Input: part model. Units: mm. Frame: model coordinates. A direction names the side the tool comes from. Give positions to 0.01 mm unless a question says otherwise; leave off trailing zeros. Loops run counter-clockwise (first coordinate to the right, second up) from the corner with the lowest first, then second, coordinate; pieces in that order, holes last. Notation, with made-up numbers: M 23.25,-15.5 L 28.25,-15.5 A20 ccw 28.25,5.5 Z; hole C -30.75,48 d11. An arc over 180 degrees is marked long. One line per item, written item: value. Start each with the question number.
(1) Pull-direction query (X, two-part tool) for faces 1 (the conical face through (26.98, -24.99, 7.22)), 2 (the flat face through (14, 23, 8)), 3 (the conical face through (13.95, 21.71, -9.38)); classes: released by +X, released by -X, zero draft, split by the parting line, or undercut.
(2) Ray query, line 1 along X through (y, z) = (-25.1, 12); line 2 along Y through (x, z) = (14.5, 13.5); line 3 along Y through (x, z) = (31, 12). Return the intervals inside material, ascending. Write a range as from..to.
(3) Section B-B on y = 0. Output: boundary loops of the cut face in (x, z).
(4) Pin query (flat end, axial travel): P1, Ø4, axis at x = 14, y = 21.5, coming from the -Z side; P2, Ø5.5, axis at y = -9.53, z = 5.5, coming from the -X side; P3, Ø4, axis at x = 6.5, y = -18, coming from the -Z side. Return the tip coordinate at first contact, or that it passes through.
(5) Section C-C on x = 22. State how many separate pieces and enclosed holes the cut face has, plus the area to 3 significant figures.
(6) Access query for faces 4 (the cylindrical face through (14.921, 20.655, -15.057)), 5 (the flat face through (16, -25, -18)), 6 (the cylindrical face through (14.1, -0.506, -22.994)). Directions: +Z, -Z, +X, -X, +Y, -Y. A direction counts if a zero-diameter tool reaches every point of the face in a straight line with its end or side. Return the directions, or none.
(7) Section A-A on z = -4. Output: boundary loops of the cut face in (x, y).
(8) Section D-D on y = -15.5. Output: boundary loops of the cut face in (x, z), plus the area to 3 significant figures.
```python
from build123d import *

# Parameters (mm, degrees)
MOTOR_SHELL_DEPTH               = 32.6
MOTOR_MOUNT_DEPTH               = 4
MOUNTING_HOLE_D                 = 3.4
MOUNTING_HOLE_CSINK_D           = 6.72
MOUNTING_HOLE_CSINK_ANGLE       = 90
HOLE_DUPLICATION_COUNT          = 3
SKETCH11_R                      = 6.5
SHAFT_BASE_CUTOUT_DEPTH         = 33.6
M3X0_5_TAPPED_HOLE1_D           = 2.5
M3X0_5_TAPPED_HOLE1_DEPTH       = 5
M3X0_5_TAPPED_HOLE1_CSINK_D     = 3.05
M3X0_5_TAPPED_HOLE1_CSINK_ANGLE = 90
M3X0_5_TAPPED_HOLE1_TIP         = 0.751075774
M3X0_5_TAPPED_HOLE2_D           = 2.5
M3X0_5_TAPPED_HOLE2_CSINK_D     = 3.05
M3X0_5_TAPPED_HOLE2_CSINK_ANGLE = 90
M3X0_5_TAPPED_HOLE3_D           = 2.5
M3X0_5_TAPPED_HOLE3_DEPTH       = 5
M3X0_5_TAPPED_HOLE3_TIP         = 0.751075774
TAP_DRILL_FOR_M3X0_5_TAP2_D     = 2.5
TAP_DRILL_FOR_M3X0_5_TAP2_DEPTH = 15
TAP_DRILL_FOR_M3X0_5_TAP2_TIP   = 0.751075774
CUT_EXTRUDE1_DEPTH              = 28.6


with BuildPart() as part:
    # Motor Shell Profile → Motor Shell (new body)
    with BuildSketch(Plane(origin=(0, 0, 0), x_dir=(0, 0, -1), z_dir=(1, 0, 0))):
        with BuildLine():
            Line((0, 22), (-16, 22))
            Line((-16, 22), (-16, 26))
            Line((-16, 26), (18, 26))
            Line((18, 26), (24.336, 9.152))
            ThreePointArc((24.336, 9.152), (25.543974558, -4.848233058), (19.290322581, -17.432253289))
            ThreePointArc((19.290322581, -17.432253289), (18.333717374, -18.988556671), (18, -20.784609691))
            Line((18, -20.784609691), (18, -29))
            Line((18, -29), (-16, -29))
            Line((-16, -29), (-16, -22))
            Line((-16, -22), (0, -22))
            ThreePointArc((0, -22), (22, 0), (0, 22))
        make_face()
    extrude(amount=MOTOR_SHELL_DEPTH)

    # Sketch3 → Motor Mount (add)
    with BuildSketch(Plane(origin=(28.6, 0, 0), x_dir=(0, 0, -1), z_dir=(1, 0, 0))):
        with BuildLine():
            Line((0, 22), (-16, 22))
            Line((-16, 22), (-16, -22))
            Line((-16, -22), (0, -22))
            ThreePointArc((0, -22), (22, 0), (0, 22))
        make_face()
    extrude(amount=MOTOR_MOUNT_DEPTH)

    # Mounting Hole (through all)
    with Locations(Plane(origin=(32.6, 0, 0), x_dir=(0, 0, -1), z_dir=(1, 0, 0))):
        with Locations((11, 0)):
            mounting_hole = CounterSinkHole(MOUNTING_HOLE_D / 2, MOUNTING_HOLE_CSINK_D / 2, counter_sink_angle=MOUNTING_HOLE_CSINK_ANGLE)

    # Hole Duplication: Mounting Hole ×3 about axis
    hole_duplication_axis = Axis((0, 0, 0), (1, 0, 0))
    for i in range(1, HOLE_DUPLICATION_COUNT):
        add(mounting_hole.rotate(hole_duplication_axis, i * 360 / HOLE_DUPLICATION_COUNT), mode=Mode.SUBTRACT)

    # Sketch11 → Shaft Base Cutout (cut, through all)
    with BuildSketch(Plane(origin=(32.6, 0, 0), x_dir=(0, 0, -1), z_dir=(1, 0, 0))):
        Circle(SKETCH11_R)
    extrude(amount=-SHAFT_BASE_CUTOUT_DEPTH, mode=Mode.SUBTRACT)

    # M3x0.5 Tapped Hole1
    with Locations(Plane(origin=(32.6, 0, 0), x_dir=(0, 0, -1), z_dir=(1, 0, 0))):
        with Locations((-7, -25), (13, -25), (-12, 18), (15, 18)):
            CounterSinkHole(M3X0_5_TAPPED_HOLE1_D / 2, M3X0_5_TAPPED_HOLE1_CSINK_D / 2, depth=M3X0_5_TAPPED_HOLE1_DEPTH, counter_sink_angle=M3X0_5_TAPPED_HOLE1_CSINK_ANGLE)
            with Locations((0, 0, -(M3X0_5_TAPPED_HOLE1_DEPTH + M3X0_5_TAPPED_HOLE1_TIP / 2))):  # 118° drill point
                Cone(0, M3X0_5_TAPPED_HOLE1_D / 2, M3X0_5_TAPPED_HOLE1_TIP, mode=Mode.SUBTRACT)

    # M3x0.5 Tapped Hole2 (through all)
    with Locations(Plane(origin=(0, 26, 0), x_dir=(1, 0, 0), z_dir=(0, 1, 0))):
        with Locations((22, -12), (8, -12), (8, 11), (22, 11)):
            CounterSinkHole(M3X0_5_TAPPED_HOLE2_D / 2, M3X0_5_TAPPED_HOLE2_CSINK_D / 2, counter_sink_angle=M3X0_5_TAPPED_HOLE2_CSINK_ANGLE)

    # M3x0.5 Tapped Hole3
    with Locations(Plane(origin=(0, 0, -18), x_dir=(-1, 0, 0), z_dir=(0, 0, -1))):
        with Locations((-24, -24.2)):
            Hole(M3X0_5_TAPPED_HOLE3_D / 2, depth=M3X0_5_TAPPED_HOLE3_DEPTH)
            with Locations((0, 0, -(M3X0_5_TAPPED_HOLE3_DEPTH + M3X0_5_TAPPED_HOLE3_TIP / 2))):  # 118° drill point
                Cone(0, M3X0_5_TAPPED_HOLE3_D / 2, M3X0_5_TAPPED_HOLE3_TIP, mode=Mode.SUBTRACT)

    # Tap Drill for M3x0.5 Tap2
    with Locations(Plane(origin=(0, 0, -25), x_dir=(1, 0, 0), z_dir=(0, 0, -1))):
        with Locations((14, -21.5)):
            Hole(TAP_DRILL_FOR_M3X0_5_TAP2_D / 2, depth=TAP_DRILL_FOR_M3X0_5_TAP2_DEPTH)
            with Locations((0, 0, -(TAP_DRILL_FOR_M3X0_5_TAP2_DEPTH + TAP_DRILL_FOR_M3X0_5_TAP2_TIP / 2))):  # 118° drill point
                Cone(0, TAP_DRILL_FOR_M3X0_5_TAP2_D / 2, TAP_DRILL_FOR_M3X0_5_TAP2_TIP, mode=Mode.SUBTRACT)

    # Sketch25 → Cut-Extrude1 (cut)
    with BuildSketch(Plane.ZY):
        with BuildLine():
            Line((0, 23), (16, 23))
            Line((16, 23), (16, -23))
            Line((16, -23), (0, -23))
            ThreePointArc((0, -23), (-23, 0), (0, 23))
        make_face()
    extrude(amount=-CUT_EXTRUDE1_DEPTH, mode=Mode.SUBTRACT)


solid = part.part
```
Output values:
1. face 1: released by +X
1. face 2: zero draft
1. face 3: undercut
2. line 1: x = 0..6.75, 9.25..20.75, 23.25..32.6
2. line 2: y = -29..-23, 23..26
2. line 3: y = -29..16.75, 19.25..26
3. outline: M 0,-26 L 32.6,-26 L 32.6,-14.36 L 30.94,-12.7 L 28.6,-12.7 L 28.6,-23 L 0,-23 Z; M 28.6,-9.3 L 30.94,-9.3 L 32.6,-7.64 L 32.6,-6.5 L 28.6,-6.5 Z; M 28.6,6.5 L 32.6,6.5 L 32.6,16 L 28.6,16 Z
4. P1: stops at z = -20.44
4. P2: stops at x = 28.6
4. P3: stops at z = -20.49
5. separate pieces: 5
5. enclosed holes: 0
5. area: 469 mm²
6. face 4: -Z
6. face 5: -Z, +X, -X, -Y
6. face 6: +Z, -X
7. outline: M 0,-29 L 32.6,-29 L 32.6,-5.12 L 28.6,-5.12 L 28.6,-22.65 L 0,-22.65 Z; M 0,22.65 L 28.6,22.65 L 28.6,5.12 L 32.6,5.12 L 32.6,26 L 0,26 Z
8. outline: M 0,-20.87 L 32.6,-20.87 L 32.6,16 L 28.6,16 L 28.6,-16.99 L 0,-16.99 Z
8. area: 259 mm²
